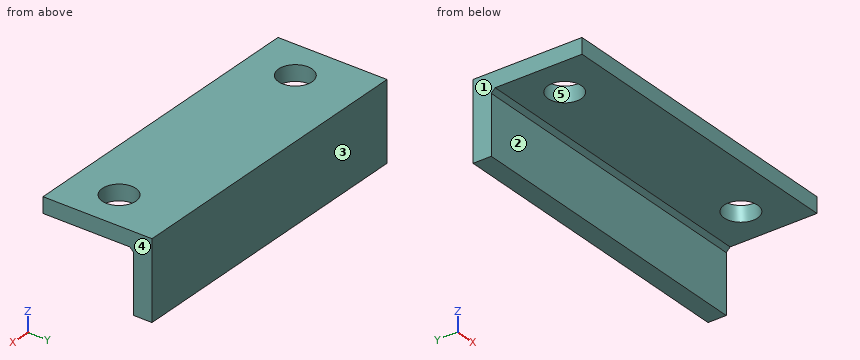
Autodesk Inventor part; units mm, degrees
ref_plane "YZ Plane" through (0, 0, 0) normal (1, 0, 0) x (0, 1, 0)
ref_plane "XZ Plane" through (0, 0, 0) normal (0, 1, 0) x (-1, 0, 0)
ref_plane "XY Plane" through (0, 0, 0) normal (0, 0, 1) x (1, 0, 0)
sketch "スケッチ1" plane through (0, 0, 0) normal (0, 0, 1) x (1, 0, 0)
  line L0 (-20, -6) -> (20, -6)
  line L1 (20, -6) -> (20, 8)
  line L2 (20, 8) -> (-20, 8)
  line L3 (-20, 8) -> (-20, -6)
  point P0 (0, 0)
  dimension "d1" = 40
  dimension "d21" = 8
  dimension "d22" = 6
  dimension "d23" = 20
extrude "押し出し1" add sketch "スケッチ1" along normal blind 2
sketch "スケッチ2" plane through (0, 0, 2) normal (0, 0, 1) x (1, 0, 0)
  line L0 (-20, -6) -> (20, -6)
  point P0 (0, 0)
  point P1 (-15, 0)
  point P2 (15, 0)
  dimension "d4" = 6
  dimension "d5" = 6
  dimension "d24" = 15
  dimension "d25" = 15
hole "穴1" at (-15, 0, 2) at (15, 0, 2) direction (0, 0, -1) diameter 4.3 end through all
sketch "スケッチ3" plane through (0, 0, 0) normal (0, 0, -1) x (-1, 0, 0)
  circle A0 centre (15, 0) radius 2.15
  circle A1 centre (-15, 0) radius 2.15
  line L0 (-20, -6) -> (-20, 8)
  line L1 (20, -6) -> (-20, -6)
  line L2 (20, 8) -> (20, -6)
  line L3 (-20, 8) -> (20, 8)
  line L4 (-20, 8) -> (20, 8)
  line L5 (20, 8) -> (20, 5.653)
  line L6 (20, 5.653) -> (-20, 5.653)
  line L7 (-20, 5.653) -> (-20, 8)
  point P0 (0, 0)
  point P1 (-20, 5.653)
  dimension "d15" = 2.347
extrude "押し出し2" add sketch "スケッチ3" along normal blind 8 contours L0 L3 L2 L6
chamfer "面取り2" distance 0.5 angle 45 1 edges at (0, 5.653, 0)
properties part number "base38" material "ABS プラスチック"
Model file for the job. Use its own axes, mm. Face numbers are marked on the shaded views. A direction names the side the tool comes from. Coordinates: 2 decimals unless noted, no trailing zeros. Write each loop counter-clockwise with the first axis right and the second up, starting at its lowest first coordinate (ties: lowest second). Pieces come first, ordered by that corner, then holes. Notation, with made-up numbers: (-32, -28) - (19, -28) arc R36 ccw to (19, 7) - close; hole circle Ø3 at (29.25, 82). An arc over 180 degrees is marked (long way). One line per question, with ' | ' between items. Start each with the question number.
Q1. Drill centre lines: line 1 (X direction, y = 0, z = 1.35); line 2 (X direction, y = -1.5, z = 1.5); line 3 (Y direction, x = 7.5, z = -3.75). Where is each one in solid material? Low to high. Write a range as [from, to].
Q2. 3-axis set-ups, long thin cutter, end or side, ignore diameter. For the marked faces 1 and 2: which of +Z, -Z, +X, -X, +Y, -Y reach the whole face in a straight line?
Q3. Cut at B-B, the plane x = -15. List the corners of the cut face in (y, z).
Q4. Pull direction Y, two halves, no side cores. Call the marked faces 3, 4 and 5: pulls with the +Y half, pulls with the -Y half, needs draft (parallel to the pull), parting line crosses it, or undercut.
Q5. Cut at D-D, the plane x = -2. List the corners of the cut face in (y, z), then the cut area to 3 significant figures.
Q6. Cut at C-C, the plane z = 1. List the corners of the cut face in (x, y), then the cut area to 3 significant figures.
Q7. Pin check, flat tips, straight feed: pin 1 (5.5 mm diameter, centred on x = -1, y = -1.5, fed in from -Z); pin 2 (1 mm diameter, centred on y = -4, z = -1, fed in from +X); pin 3 (1 mm diameter, centred on x = 3.5, z = -6, fed in from -Y). Stop position of each tip, or through.
Q8. Cut at A-A, the plane y = 0. List the corners of the cut face in (x, z).
Answer below:
1) line 1: [-20, -17.15], [-12.85, 12.85], [17.15, 20] | line 2: [-20, -16.54], [-13.46, 13.46], [16.54, 20] | line 3: [5.65, 8]
2) face 1: +Z, -Z, -X, +Y, -Y | face 2: -Z, +X, -X, -Y
3) outline: (-6, 0) - (-2.15, 0) - (-2.15, 2) - (-6, 2) - close; (2.15, 0) - (5.15, 0) - (5.65, -0.5) - (5.65, -8) - (8, -8) - (8, 2) - (2.15, 2) - close
4) face 3: pulls with the +Y half | face 4: needs draft | face 5: undercut
5) outline: (-6, 0) - (5.15, 0) - (5.65, -0.5) - (5.65, -8) - (8, -8) - (8, 2) - (-6, 2) - close | area: 46.9 mm^2
6) outline: (-20, -6) - (20, -6) - (20, 8) - (-20, 8) - close; hole circle Ø4.3 at (-15, 0); hole circle Ø4.3 at (15, 0) | area: 531 mm^2
7) pin 1: z = 0 | pin 2: through | pin 3: y = 5.65
8) outline: (-20, 0) - (-17.15, 0) - (-17.15, 2) - (-20, 2) - close; (-12.85, 0) - (12.85, 0) - (12.85, 2) - (-12.85, 2) - close; (17.15, 0) - (20, 0) - (20, 2) - (17.15, 2) - close
